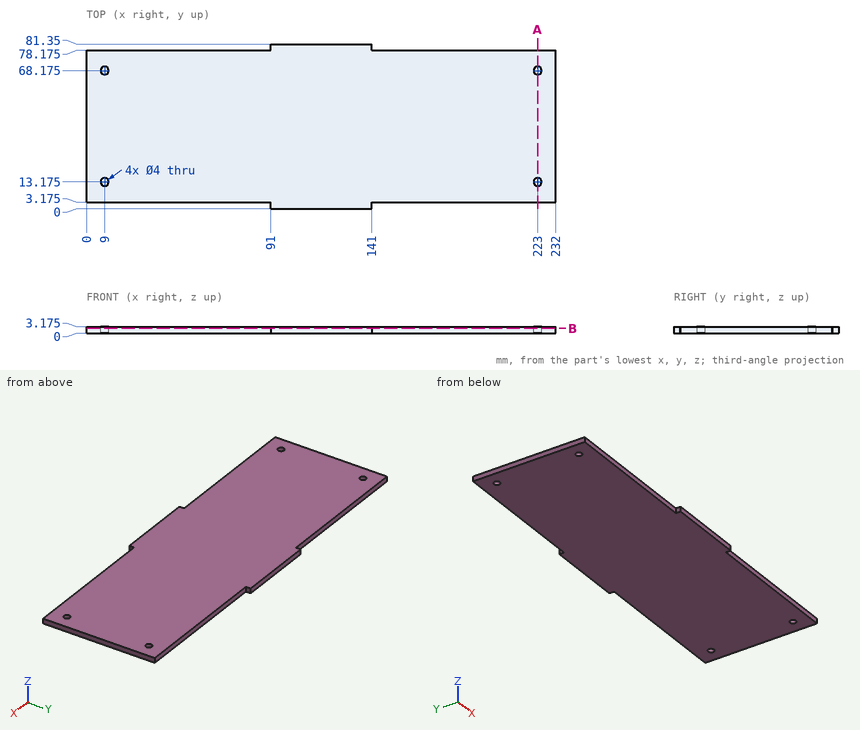
Geometry check sheet. Reference: drawing and pictorial views, mm from the part's lowest x, y, z. Round coordinates to 2 decimals unless told otherwise and drop trailing zeros. Write each loop counter-clockwise with the first axis right and the second up, starting at its lowest first coordinate (ties: lowest second). Pieces come first, ordered by that corner, then holes. Notation, with made-up numbers: (46.25, 47.25) -> (50.25, 47.25) arc R12 ccw to (50.25, 53.25) -> close; hole circle Ø5 at (74, 56.5). An arc over 180 degrees is marked (long way). Answer as CSV lines item,"result". Start each with the question number.
1) Material ranges on line 1 (Y direction, x = 223, z = 1.9) (3 decimals); line 2 (X direction, y = 68, z = 0.55); line 3 (Y direction, x = 221.5, z = 2.95) (3 decimals), recorded low to high. Write a range as from..to.
2) Section check A-A on x = 223. Enter the section's corners in (y, z) (3 decimals), and give its area (3 significant figures).
3) Go/stop test with flat-tipped pins: P1, Ø1.6, axis at y = 2, z = 2.5, coming from the +X side; P2, Ø3.5, axis at x = 9, y = 68.175, coming from the -Z side; P3, Ø1, axis at y = 2, z = 1, coming from the -X side; P4, Ø1.6, axis at x = 180.5, z = 1.5, coming from the -Y side (3 decimals). Record where each tip stops, or that it passes through.
4) Section check B-B on z = 2.35. Enter the section's corners in (x, y) (3 decimals), and give its area (3 significant figures).
Found:
1,line 1,"y = 3.175..11.175, 15.175..66.175, 70.175..78.175"
1,line 2,"x = 0..7.01, 10.99..221.01, 224.99..232"
1,line 3,"y = 3.175..11.852, 14.498..66.852, 69.498..78.175"
2,outline,"(3.175, 0) -> (11.175, 0) -> (11.175, 3.175) -> (3.175, 3.175) -> close; (15.175, 0) -> (66.175, 0) -> (66.175, 3.175) -> (15.175, 3.175) -> close; (70.175, 0) -> (78.175, 0) -> (78.175, 3.175) -> (70.175, 3.175) -> close"
2,area,"213 mm^2"
3,P1,"stops at x = 141"
3,P2,"passes through"
3,P3,"stops at x = 91"
3,P4,"stops at y = 3.175"
4,outline,"(0, 3.175) -> (91, 3.175) -> (91, 0) -> (141, 0) -> (141, 3.175) -> (232, 3.175) -> (232, 78.175) -> (141, 78.175) -> (141, 81.35) -> (91, 81.35) -> (91, 78.175) -> (0, 78.175) -> close; hole circle Ø4 at (9, 13.175); hole circle Ø4 at (9, 68.175); hole circle Ø4 at (223, 13.175); hole circle Ø4 at (223, 68.175)"
4,area,"17,700 mm^2"
